Verification items for the finished model (mm, model axes). A direction names the side the tool comes from. Give positions to 0.01 mm unless a question says otherwise; leave off trailing zeros. Write each loop counter-clockwise with the first axis right and the second up, starting at its lowest first coordinate (ties: lowest second). Pieces come first, ordered by that corner, then holes. Notation, with made-up numbers: (49.5, -28.75) -> (79.5, -28.75) arc R19 cw to (79.5, -19.75) -> close; hole circle Ø4 at (-17.75, 46). An arc over 180 degrees is marked (long way). Answer as CSV lines item,"result".
```python
from build123d import *

# Parameters (mm, degrees)
F0_W     = 50
F0_H     = 12
F0_R     = 2.5
F1_DEPTH = 12
F2_R     = 5
F4_DEPTH = 25


with BuildPart() as f1:
    # F0 (on Front) → F1 (new body)
    with BuildSketch(Plane.XZ):
        Rectangle(F0_W, F0_H)
        with Locations((-17.5, 0)):
            Circle(F0_R, mode=Mode.SUBTRACT)
        with Locations((17.5, 0)):
            Circle(F0_R, mode=Mode.SUBTRACT)
    extrude(amount=F1_DEPTH)

    # F2
    f2_edges = [f1.edges().sort_by_distance(p)[0] for p in [
        (-25, -6, 6),
        (25, -6, 6),
        (25, -6, -6),
        (-25, -6, -6),
    ]]
    fillet(f2_edges, radius=F2_R)

    # F3 (on face) → F4 (cut)
    with BuildSketch(Plane.XZ.offset(12)):
        Polygon((2, -4), (0, -6), (17.5, -6), (15.5, -4), align=None)
        Polygon((-17.5, -6), (0, -6), (-2, -4), (-15.5, -4), align=None)
        with BuildLine():
            Line((19.5, -4), (17.5, -6))
            Line((17.5, -6), (20, -6))
            ThreePointArc((20, -6), (22.236068, -5.472136), (24, -4))
            Line((24, -4), (19.5, -4))
        make_face()
        with BuildLine():
            Line((-20, -6), (-17.5, -6))
            Line((-17.5, -6), (-19.5, -4))
            Line((-19.5, -4), (-24, -4))
            ThreePointArc((-24, -4), (-22.236068, -5.472136), (-20, -6))
        make_face()
    extrude(amount=-F4_DEPTH, mode=Mode.SUBTRACT)


solid = f1.part
```
1) Scan lines: line 1 along X through (y, z) = (-10.25, -1); line 2 along X through (y, z) = (-2, -4.75); line 3 along Z through (x, y) = (7, -8.5). Record each from-to range of solid material in increasing order.
Reported:
line 1,"-25 to -19.79, -15.21 to 15.21, 19.79 to 25"
line 2,"-18.75 to -16.25, -1.25 to 1.25, 16.25 to 18.75"
line 3,"-4 to 6"
2) Draft check along X on faces 1 (the cylindrical face through (15, -6, 0)), 2 (the flat face through (-25, -6, 0)), 3 (the flat face through (-22, -6, -4)), 4 (the flat face through (9, -6, -4)). Enter one of: +X half, -X half, draft (parallel to the pull), parting line (faces both ways), or undercut.
Reported:
face 1,"undercut"
face 2,"-X half"
face 3,"draft"
face 4,"undercut"
3) Section check D-D (z = -3). Record the boundary of the cut face in (x, y).
Reported:
outline,"(-24.58, -12) -> (24.58, -12) -> (24.58, 0) -> (-24.58, 0) -> close"
4) Section check C-C (x = -3.5). Record the boundary of the cut face in (y, z), and give its area (3 significant figures).
Reported:
outline,"(-12, -4) -> (0, -4) -> (0, 6) -> (-12, 6) -> close"
area,"120 mm²"
5) Depth check by flat-ended pin: pin 1 (2 mm diameter, centred on x = 17, z = 0.5, fed in from -Y); pin 2 (3.5 mm diameter, centred on x = -8, y = -7.5, fed in from -Z); pin 3 (1 mm diameter, centred on y = -9, z = 1.5, fed in from +X); pin 4 (5 mm diameter, centred on x = -21, y = -8.5, fed in from -Z). Enter the tip coordinate at first touch or a pass-through.
Reported:
pin 1,"through"
pin 2,"z = -4"
pin 3,"x = 25"
pin 4,"z = -5"
6) Tool access check on faces 5 (the flat face through (16.5, -6.1, -5)), 6 (the flat face through (0, -12, 0)). Record the directions out of +Z, -Z, +X, -X, +Y, -Y that give a thin tool (end or side, any length) a straight path to the whole face; none if there is none.
Reported:
face 5,"-Z, +Y, -Y"
face 6,"+Z, -Z, +X, -X, -Y"
7) Section check B-B (z = 0). Record the boundary of the cut face in (x, y), and give its area (3 significant figures).
Reported:
outline,"(-25, -12) -> (-20, -12) -> (-20, 0) -> (-25, 0) -> close; (-15, -12) -> (15, -12) -> (15, 0) -> (-15, 0) -> close; (20, -12) -> (25, -12) -> (25, 0) -> (20, 0) -> close"
area,"480 mm²"
8) Section check A-A (y = -7.5). Record the boundary of the cut face in (x, z).
Reported:
outline,"(-25, -1) arc R5 ccw to (-24, -4) -> (-19.5, -4) -> (-17.5, -6) -> (-15.5, -4) -> (-2, -4) -> (0, -6) -> (2, -4) -> (15.5, -4) -> (17.5, -6) -> (19.5, -4) -> (24, -4) arc R5 ccw to (25, -1) -> (25, 1) arc R5 ccw to (20, 6) -> (-20, 6) arc R5 ccw to (-25, 1) -> close; hole circle Ø5 at (-17.5, 0); hole circle Ø5 at (17.5, 0)"
